Input: dimensioned drawing with shaded views. Units: mm. Origin: part minimum x, y, z. A direction names the side the tool comes from. Coordinates: 2 decimals unless noted, no trailing zeros. Write each loop counter-clockwise with the first axis right and the second up, starting at its lowest first coordinate (ties: lowest second). Pieces come first, ordered by that corner, then holes. Notation, with made-up numbers: M -28.75,22 L 3.25,22 A24 ccw 3.25,59 Z; hole C 18,18.5 d5. An arc over 180 degrees is marked long. Write each question's results on one line, items separated by ' | '. Start each with the question number.
1. Section query C-C, the plane y = 7. Output: boundary loops of the cut face in (x, z).
2. First-contact query: pin 1 (0.8 mm diameter, centred on y = 5.5, z = 7.5, fed in from -X); pin 2 (2.5 mm diameter, centred on x = 5, y = 5.77, fed in from -Z); pin 3 (2.5 mm diameter, centred on x = 6, y = 6.5, fed in from -Z); pin 4 (5 mm diameter, centred on x = 8, z = 7.5, fed in from -Y). Flat tips, straight axial feed; report the tip coordinate or a pass-through.
3. Section query D-D, the plane z = 4.25. Output: boundary loops of the cut face in (x, y) (1 decimal).
4. Section query A-A, the plane x = 6. Output: boundary loops of the cut face in (y, z) (1 decimal).
5. Pull-direction query (X, two-part tool) for the marked faces 1, 2 and 3; classes: +X half, -X half, draft (parallel to the pull), parting line (faces both ways), or undercut.
6. Ray query, probe 1 along X at (y, z) = (5.75, 3); probe 2 along Z at (x, y) = (7.5, 4.5); probe 3 along X at (y, z) = (9, 5.25) (1 decimal). Return the intervals inside material, ascending.
7. Set-up query: the marked faces 4 and 5. Return all of +Z, -Z, +X, -X, +Y, -Y with unobstructed straight access to the full face (end or side cutting, diameter ignored); none if empty.
8. Section query B-B, the plane z = 2.5. Output: boundary loops of the cut face in (x, y).
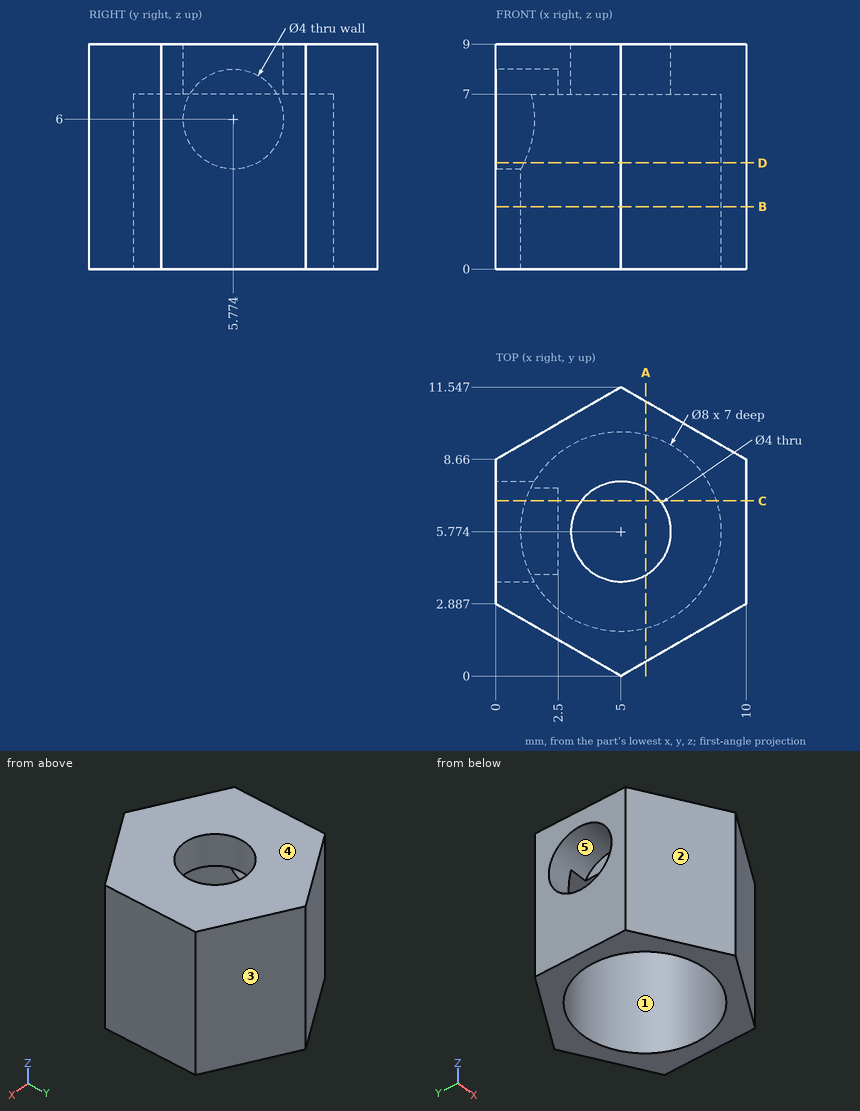
Answer:
1) outline: M 0,0 L 1.19,0 L 1.19,4.42 L 0,4.42 Z; M 0,7.58 L 2.5,7.58 L 2.5,7 L 3.42,7 L 3.42,9 L 0,9 Z; M 6.58,7 L 8.81,7 L 8.81,0 L 10,0 L 10,9 L 6.58,9 Z
2) pin 1: x = 2.5 | pin 2: through | pin 3: z = 7 | pin 4: y = 0.29
3) outline: M 0,2.9 L 5,0 L 10,2.9 L 10,8.7 L 5,11.5 L 0,8.7 L 0,6.7 L 1.1,6.7 A4 cw long 1.1,4.8 L 0,4.8 Z
4) outline: M 0.6,0 L 1.9,0 L 1.9,7 L 4,7 L 4,9 L 0.6,9 Z; M 7.5,7 L 9.6,7 L 9.6,0 L 11,0 L 11,9 L 7.5,9 Z
5) face 1: undercut | face 2: -X half | face 3: +X half
6) probe 1: 0 to 1, 9 to 10 | probe 2: 7 to 9 | probe 3: 0.6 to 2.6, 7.4 to 9.4
7) face 4: +Z, +X, -X, +Y, -Y | face 5: -X
8) outline: M 0,2.89 L 5,0 L 10,2.89 L 10,8.66 L 5,11.55 L 0,8.66 Z; hole C 5,5.77 d8
